from build123d import *

# Parameters (mm, degrees)
F1_DEPTH    = 8.2
F2_DEPTH    = 1.2
F3_DEPTH    = 2
F4_R        = 0.4
F5_T1_DEPTH = 2
F5_T3_DEPTH = 4


# Not quite as in the source:
# - a fillet or chamfer that OpenCascade refuses, or shapes differently, is made with other operations: its cross-section is extruded or revolved along the edge and cut away or added
# - a feature names something its author has since deleted; it is built from what else it names


with BuildPart() as f1:
    # F0 (on Top) → F1 (new body)
    with BuildSketch(Plane.XY):
        with BuildLine():
            Line((-5.7662812973, -3), (-7.0915442606, -3))
            ThreePointArc((-7.0915442606, -3), (-6.7991383758, -3.6140997975), (-6.4536811201, -4.2))
            ThreePointArc((-6.4536811201, -4.2), (7.7, 0), (-6.4536811201, 4.2))
            ThreePointArc((-6.4536811201, 4.2), (-6.7991383758, 3.6140997975), (-7.0915442606, 3))
            Line((-7.0915442606, 3), (-5.7662812973, 3))
            ThreePointArc((-5.7662812973, 3), (-0.2675331935, 6.4944919732), (5.5, 3.4641016151))
            ThreePointArc((5.5, 3.4641016151), (6.5, 0), (5.5, -3.4641016151))
            ThreePointArc((5.5, -3.4641016151), (-0.2675331935, -6.4944919732), (-5.7662812973, -3))
        make_face()
        with BuildLine():
            Line((5.5, 3.4641016151), (5.5, -3.4641016151))
            ThreePointArc((5.5, -3.4641016151), (6.5, 0), (5.5, 3.4641016151))
        make_face()
    extrude(amount=F1_DEPTH)

    # F0 (on Top) → F2 (join)
    with BuildSketch(Plane.XY):
        with BuildLine():
            Line((0, -3), (-5.7662812973, -3))
            ThreePointArc((-5.7662812973, -3), (-0.2675331935, -6.4944919732), (5.5, -3.4641016151))
            Line((5.5, -3.4641016151), (5.5, 3.4641016151))
            ThreePointArc((5.5, 3.4641016151), (-0.2675331935, 6.4944919732), (-5.7662812973, 3))
            Line((-5.7662812973, 3), (0, 3))
            ThreePointArc((0, 3), (3, 0), (0, -3))
        make_face()
        with BuildLine():
            Line((5.5, 3.4641016151), (5.5, -3.4641016151))
            ThreePointArc((5.5, -3.4641016151), (6.5, 0), (5.5, 3.4641016151))
        make_face()
    extrude(amount=F2_DEPTH)

    # F0 (on Top) → F3 (join)
    with BuildSketch(Plane.XY):
        with BuildLine():
            ThreePointArc((-7.0915442606, 3), (-6.7991383758, 3.6140997975), (-6.4536811201, 4.2))
            Line((-6.4536811201, 4.2), (-7.9657880694, 4.2))
            Line((-7.9657880694, 4.2), (-7.9657880694, 6.8))
            Line((-7.9657880694, 6.8), (-6.7657880694, 6.8))
            Line((-6.7657880694, 6.8), (-6.7657880694, 8))
            Line((-6.7657880694, 8), (-7.9657880694, 8))
            Line((-7.9657880694, 8), (-9.1657880694, 8))
            Line((-9.1657880694, 8), (-9.1657880694, 3))
            Line((-9.1657880694, 3), (-7.0915442606, 3))
        make_face()
        with BuildLine():
            ThreePointArc((-6.4536811201, -4.2), (-6.7991383758, -3.6140997975), (-7.0915442606, -3))
            Line((-7.0915442606, -3), (-9.1657880694, -3))
            Line((-9.1657880694, -3), (-9.1657880694, -8))
            Line((-9.1657880694, -8), (-7.9657880694, -8))
            Line((-7.9657880694, -8), (-6.7657880694, -8))
            Line((-6.7657880694, -8), (-6.7657880694, -6.8))
            Line((-6.7657880694, -6.8), (-7.9657880694, -6.8))
            Line((-7.9657880694, -6.8), (-7.9657880694, -4.2))
            Line((-7.9657880694, -4.2), (-6.4536811201, -4.2))
        make_face()
    extrude(amount=F3_DEPTH)

    # F4
    f4_edges = [f1.edges().sort_by_distance(p)[0] for p in [
        (-7.091544, 3, 5.1),
        (-7.091544, -3, 5.1),
    ]]
    fillet(f4_edges, radius=F4_R)

    # F5: fillet of radius 0.4 on 14 edges, made by hand

    # F5_s2 → F5_t1 (join)
    with BuildSketch(Plane.XY):
        with BuildLine():
            ThreePointArc((-7.5657880694, 4.2), (-7.8486307818, 4.3171572875), (-7.9657880694, 4.6))
            Line((-7.9657880694, 4.6), (-7.9657880694, 4.2))
            Line((-7.9657880694, 4.2), (-7.5657880694, 4.2))
        make_face()
        with BuildLine():
            ThreePointArc((-6.3378446378, 4.3728395062), (-6.48115887, 4.2458360567), (-6.6670833203, 4.2))
            Line((-6.6670833203, 4.2), (-6.4536811201, 4.2))
            ThreePointArc((-6.4536811201, 4.2), (-6.3963467056, 4.2868110318), (-6.3378446378, 4.3728395062))
        make_face()
        with BuildLine():
            ThreePointArc((-6.3378446378, -4.3728395062), (-6.48115887, -4.2458360567), (-6.6670833203, -4.2))
            Line((-6.6670833203, -4.2), (-6.4536811201, -4.2))
            ThreePointArc((-6.4536811201, -4.2), (-6.3963467056, -4.2868110318), (-6.3378446378, -4.3728395062))
        make_face()
        with BuildLine():
            ThreePointArc((-7.5657880694, -4.2), (-7.8486307818, -4.3171572875), (-7.9657880694, -4.6))
            Line((-7.9657880694, -4.6), (-7.9657880694, -4.2))
            Line((-7.9657880694, -4.2), (-7.5657880694, -4.2))
        make_face()
        with BuildLine():
            ThreePointArc((-7.9657880694, -6.4), (-7.8486307818, -6.6828427125), (-7.5657880694, -6.8))
            Line((-7.5657880694, -6.8), (-7.9657880694, -6.8))
            Line((-7.9657880694, -6.8), (-7.9657880694, -6.4))
        make_face()
        with BuildLine():
            ThreePointArc((-7.9657880694, 6.4), (-7.8486307818, 6.6828427125), (-7.5657880694, 6.8))
            Line((-7.5657880694, 6.8), (-7.9657880694, 6.8))
            Line((-7.9657880694, 6.8), (-7.9657880694, 6.4))
        make_face()
    extrude(amount=F5_T1_DEPTH)

    # F5_s4 → F5_t3 (cut)
    with BuildSketch(Plane.XY.offset(-1)):
        with BuildLine():
            ThreePointArc((-8.7657880694, -8), (-9.0486307818, -7.8828427125), (-9.1657880694, -7.6))
            Line((-9.1657880694, -7.6), (-9.1657880694, -8))
            Line((-9.1657880694, -8), (-8.7657880694, -8))
        make_face()
        with BuildLine():
            ThreePointArc((-8.7657880694, -3), (-9.0486307818, -3.1171572875), (-9.1657880694, -3.4))
            Line((-9.1657880694, -3.4), (-9.1657880694, -3))
            Line((-9.1657880694, -3), (-8.7657880694, -3))
        make_face()
        with BuildLine():
            ThreePointArc((-8.7657880694, 3), (-9.0486307818, 3.1171572875), (-9.1657880694, 3.4))
            Line((-9.1657880694, 3.4), (-9.1657880694, 3))
            Line((-9.1657880694, 3), (-8.7657880694, 3))
        make_face()
        with BuildLine():
            ThreePointArc((-8.7657880694, 8), (-9.0486307818, 7.8828427125), (-9.1657880694, 7.6))
            Line((-9.1657880694, 7.6), (-9.1657880694, 8))
            Line((-9.1657880694, 8), (-8.7657880694, 8))
        make_face()
        with BuildLine():
            ThreePointArc((-7.1657880694, 6.8), (-6.8829453569, 6.9171572875), (-6.7657880694, 7.2))
            Line((-6.7657880694, 7.2), (-6.7657880694, 6.8))
            Line((-6.7657880694, 6.8), (-7.1657880694, 6.8))
        make_face()
        with BuildLine():
            ThreePointArc((-6.7657880694, -7.6), (-6.8829453569, -7.8828427125), (-7.1657880694, -8))
            Line((-7.1657880694, -8), (-6.7657880694, -8))
            Line((-6.7657880694, -8), (-6.7657880694, -7.6))
        make_face()
        with BuildLine():
            ThreePointArc((-7.1657880694, -6.8), (-6.8829453569, -6.9171572875), (-6.7657880694, -7.2))
            Line((-6.7657880694, -7.2), (-6.7657880694, -6.8))
            Line((-6.7657880694, -6.8), (-7.1657880694, -6.8))
        make_face()
        with BuildLine():
            ThreePointArc((-6.7657880694, 7.6), (-6.8829453569, 7.8828427125), (-7.1657880694, 8))
            Line((-7.1657880694, 8), (-6.7657880694, 8))
            Line((-6.7657880694, 8), (-6.7657880694, 7.6))
        make_face()
    extrude(amount=F5_T3_DEPTH, mode=Mode.SUBTRACT)


solid = f1.part
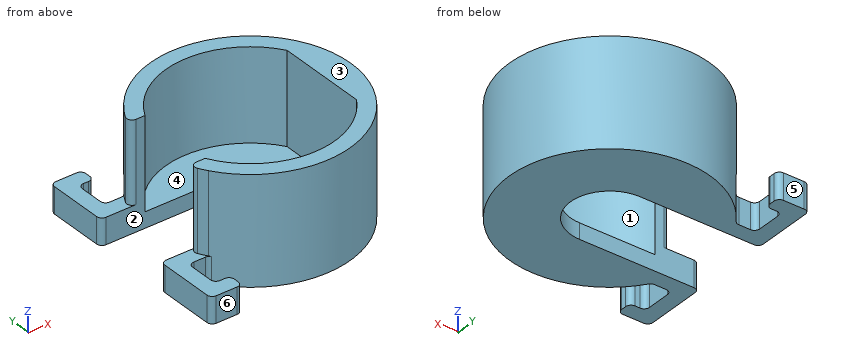
Design review of the part built by this model. Coordinates are the model's own, in mm. Face numbers are marked on the shaded views. A direction names the side the tool comes from. Round coordinates to 2 decimals unless told otherwise and drop trailing zeros. Write each loop counter-clockwise with the first axis right and the second up, starting at its lowest first coordinate (ties: lowest second). Pieces come first, ordered by that corner, then holes. Notation, with made-up numbers: (69, -7.75) -> (78, -7.75) arc R32 cw to (78, 23.25) -> close; hole circle Ø8 at (-36, 24.25). An arc over 180 degrees is marked (long way). One line per item, written item: value. Start each with the question number.
Q1. Tool access review of the marked faces 1, 2 and 3: name each direction out of +Z, -Z, +X, -X, +Y, -Y from which nothing blocks a thin tool from reaching the whole face with its end or side.
Q2. Add section D-D (y = 1.25). Give the boundary of the cut face in (x, z), then the cut area to 3 significant figures.
Q3. Insertion check: P1, Ø2.5, axis at x = -6, z = 5.5, coming from the +Y side; P2, Ø2, axis at x = -5, z = 3, coming from the -Y side; P3, Ø0.9, axis at y = 6, z = 1, coming from the +X side. Each pin has a flat end and moves straight along its axis. Give the tip position at first contact, or say it passes through.
Q4. To check wall thickness, follow probe 1 along X at (y, z) = (-5, 1.25); probe 2 along Y at (x, z) = (0.25, 7.75); probe 3 along X at (y, z) = (4.5, 5.75). State the ranges of each line that lie inside material, in increasing order.
Q5. The part is to be moulded in two halves that separate along Y. For the marked faces 4, 5 and 6, say which applies: pulls with the +Y half, pulls with the -Y half, needs draft (parallel to the pull), parting line crosses it, or undercut.
Q6. Add section C-C (y = -5.75). Give the boundary of the cut face in (x, z), then the cut area to 3 significant figures.
Q7. Add section B-B (x = -6). Give the boundary of the cut face in (y, z), then the cut area to 3 significant figures.
Response:
1. face 1: +Z
1. face 2: +Z, -Z, -X
1. face 3: +Z, +X, -X, +Y, -Y
2. outline: (2.73, 0) -> (7.6, 0) -> (7.6, 8.2) -> (5.5, 8.2) -> (5.5, 1.2) -> (2.73, 1.2) -> close
2. area: 20.5 mm^2
3. P1: stops at y = 6.06
3. P2: stops at y = -6.58
3. P3: stops at x = 5.34
4. probe 1: x = -9.17 to -7.97, -5.86 to -4.15, 4.15 to 5.86
4. probe 2: y = -7.7 to -6.5, 6.5 to 7.7
4. probe 3: x = -6.25 to -4.69, 4.69 to 6.25
5. face 4: undercut
5. face 5: pulls with the +Y half
5. face 6: pulls with the -Y half
6. outline: (-9.17, 0) -> (-7.97, 0) -> (-7.97, 2) -> (-9.17, 2) -> close; (-5.12, 0) -> (5.12, 0) -> (5.12, 8.2) -> (3.03, 8.2) -> (3.03, 1.2) -> (-3.03, 1.2) -> (-3.03, 8.2) -> (-5.12, 8.2) -> close
6. area: 44.0 mm^2
7. outline: (-4.83, 0) -> (-3, 0) -> (-3, 8.2) -> (-4.83, 8.2) -> close; (3, 0) -> (4.83, 0) -> (4.83, 8.2) -> (3, 8.2) -> close
7. area: 29.9 mm^2
